Answer from the drawing. Dimensions are ordinates in mm from the lowest x, y and z of the part. Coordinates: 2 decimals unless noted, no trailing zeros. Order: outer loops, then holes, each group sorted by start corner. A loop starts at its lowest first (then second) coordinate and runs counter-clockwise, first axis right, second up. Notation, with made-up numbers: (23, 1) -> (35, 1) arc R18 cw to (35, 13) -> close; hole circle Ø2 at (82.5, -5.5). An arc over 180 degrees is marked (long way). Answer in a Markdown table with one row per item.
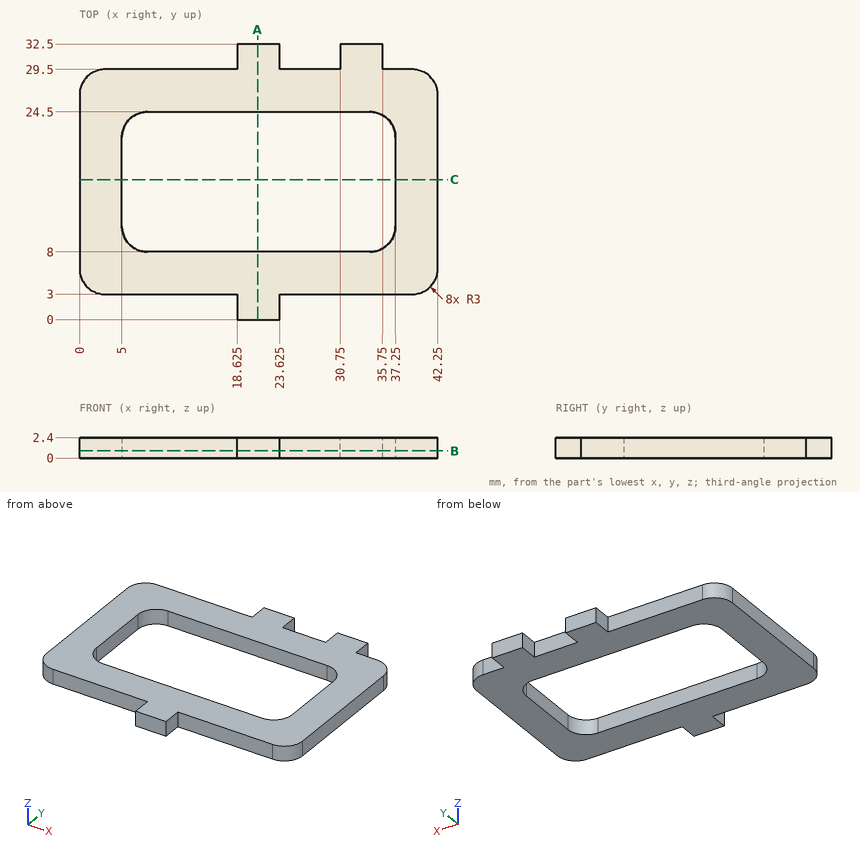
(1) A cutting plane is placed at A-A, the plane x = 21. Determine the outline of the cut face in (y, z), then the cut area to 3 significant figures.
Check values:
| item | result |
|---|---|
| outline | (0, 0) -> (8, 0) -> (8, 2.4) -> (0, 2.4) -> close; (24.5, 0) -> (32.5, 0) -> (32.5, 2.4) -> (24.5, 2.4) -> close |
| area | 38.4 mm² |
(2) A cutting plane is placed at B-B, the plane z = 0.85. Determine the outline of the cut face in (x, y) (3 decimals).
Check values:
| item | result |
|---|---|
| outline | (0, 6) arc R3 ccw to (3, 3) -> (18.625, 3) -> (18.625, 0) -> (23.625, 0) -> (23.625, 3) -> (39.25, 3) arc R3 ccw to (42.25, 6) -> (42.25, 26.5) arc R3 ccw to (39.25, 29.5) -> (35.75, 29.5) -> (35.75, 32.5) -> (30.75, 32.5) -> (30.75, 29.5) -> (23.625, 29.5) -> (23.625, 32.5) -> (18.625, 32.5) -> (18.625, 29.5) -> (3, 29.5) arc R3 ccw to (0, 26.5) -> close; hole (5, 11) arc R3 ccw to (8, 8) -> (34.25, 8) arc R3 ccw to (37.25, 11) -> (37.25, 21.5) arc R3 ccw to (34.25, 24.5) -> (8, 24.5) arc R3 ccw to (5, 21.5) -> close |
(3) A cutting plane is placed at C-C, the plane y = 16.5. Determine the outline of the cut face in (x, z).
Check values:
| item | result |
|---|---|
| outline | (0, 0) -> (5, 0) -> (5, 2.4) -> (0, 2.4) -> close; (37.25, 0) -> (42.25, 0) -> (42.25, 2.4) -> (37.25, 2.4) -> close |
(4) Find the intervals of material crossed by line 1 along Y through (x, z) = (20, 1.35); line 2 along Y through (x, z) = (25.5, 2.15); line 3 along X through (y, z) = (13.5, 0.1), in increasing order. Write a range as from..to.
Check values:
| item | result |
|---|---|
| line 1 | 0..8, 24.5..32.5 |
| line 2 | 3..8, 24.5..29.5 |
| line 3 | 0..5, 37.25..42.25 |
(5) Flat-ended cylindrical pins translate along their axes: pin 1 (8 mm diameter, centred on x = 25.5, y = 8, fed in from -Z); pin 2 (1.2 mm diameter, centred on x = 37.5, z = 1, fed in from +Y); pin 3 (10 mm diameter, centred on x = 17.5, y = 14.5, fed in from +Z); pin 4 (0.7 mm diameter, centred on y = 1.5, z = 1.5, fed in from +X) (3 decimals). Find the tip coordinate at first contact, or state that the pin passes through.
Check values:
| item | result |
|---|---|
| pin 1 | z = 0 |
| pin 2 | y = 29.5 |
| pin 3 | through |
| pin 4 | x = 23.625 |
